Study the drawing (mm; zero at the part's minimum x, y, z) and answer. A direction names the side the tool comes from. Coordinates: 2 decimals unless noted, no trailing zeros. Loops run counter-clockwise (first coordinate to the right, second up) from the corner with the lowest first, then second, coordinate; pieces in that order, holes last. Notation, with made-up numbers: M 81,78 L 102,78 A10 ccw 102,88 Z; hole C 69.5,-22 d11. An arc over 180 degrees is marked long. Use one line per item in the form item = value. Start each with the question number.
1. Find the intervals of material crossed by probe 1 along Y at (x, z) = (105.5, 62.5); probe 2 along Y at (x, z) = (93, 17.5); probe 3 along X at (y, z) = (299, 33.5), in increasing order. Write a range as [from, to].
2. The part is cut by section D-D (z = 13). Give the vertices of the cut face in (x, y).
3. The part is cut by section A-A (z = 37.5). Give the vertices of the cut face in (x, y).
4. The part is cut by section C-C (y = 37.5). Give the vertices of the cut face in (x, z), plus the area to 3 significant figures.
5. Flat-ended cylindrical pins translate along their axes: pin 1 (5 mm diameter, centred on x = 58, y = 368, fed in from +Z); pin 2 (3 mm diameter, centred on y = 398, z = 53.5, fed in from -X); pin 3 (3 mm diameter, centred on y = 121.5, z = 13, fed in from +X); pin 4 (4 mm diameter, centred on y = 154, z = 39, fed in from -X). Find the tip coordinate at first contact, or state that the pin passes through.
6. The part is cut by section B-B (x = 103.5). Give the vertices of the cut face in (y, z), plus the area to 3 significant figures.
7. A tool of negligible diameter and unlimited length cuts with its end or side. For the marked faces 1, 2 and 3, from which of +Z, -Z, +X, -X, +Y, -Y can it reach the whole face along a straight path? Write none if from no direction.
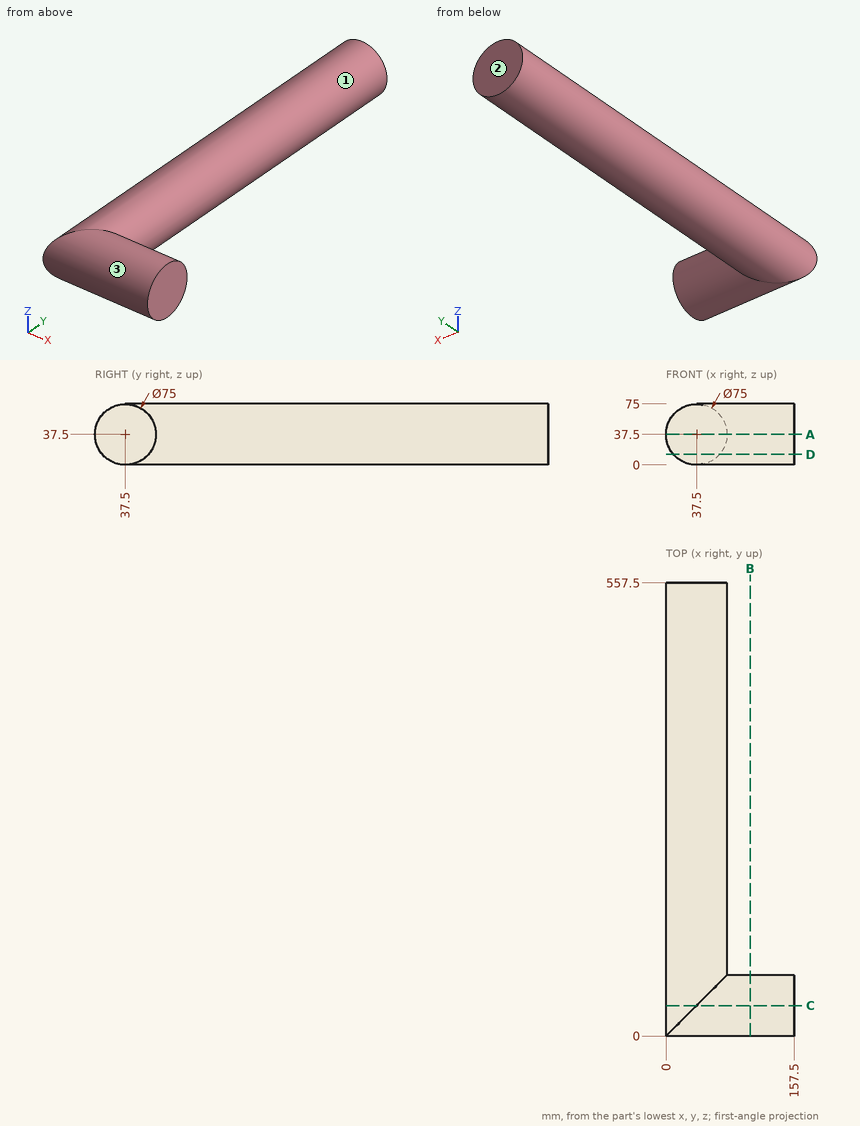
Computed values:
q1.probe_1 = [9.55, 65.45]
q1.probe_2 = [5.78, 69.22]
q1.probe_3 = [0.21, 74.79]
q2.outline = M 9.11,9.11 L 157.5,9.11 L 157.5,65.89 L 65.89,65.89 L 65.89,557.5 L 9.11,557.5 Z
q3.outline = M 0,0 L 157.5,0 L 157.5,75 L 75,75 L 75,557.5 L 0,557.5 Z
q4.outline = M 37.5,0 L 157.5,0 L 157.5,75 L 37.5,75 A37.5 ccw Z
q4.area = 11,200 mm²
q5.pin_1 = 70.4
q5.pin_2 = 2.92
q5.pin_3 = 67.12
q5.pin_4 = 0
q6.outline = C 37.5,37.5 d75
q6.area = 4,420 mm²
q7.face_1 = +Y
q7.face_2 = +Z, -Z, +X, -X, +Y
q7.face_3 = +X
